from build123d import *

# Parameters (mm, degrees)
SKETCH1_W           = 304.8
SKETCH1_H           = 304.8
SKETCH1_R           = 6.3627
SKETCH1_R_2         = 1.778
SKETCH1_R_3         = 1.524
SKETCH1_R_4         = 1.190625
SKETCH1_W_2         = 10.0000054
SKETCH1_H_2         = 18.9999874
SKETCH1_W_3         = 71.12
SKETCH1_H_3         = 18.415
BOSS_EXTRUDE1_DEPTH = 2.54


with BuildPart() as part:
    # Sketch1 → Boss-Extrude1 (new body)
    with BuildSketch(Plane(origin=(0, 0, 0), x_dir=(1, 0, 0), z_dir=(0, 1, 0))):
        Rectangle(SKETCH1_W, SKETCH1_H)
        with Locations(Location((-133.35, 133.35, 0), (0, 0, 270))):
            Circle(SKETCH1_R, mode=Mode.SUBTRACT)
        with Locations(Location((-114.3, 133.35, 0), (0, 0, 270))):
            Circle(SKETCH1_R, mode=Mode.SUBTRACT)
        with Locations(Location((-95.25, 133.35, 0), (0, 0, 270))):
            Circle(SKETCH1_R, mode=Mode.SUBTRACT)
        with Locations(Location((-76.2, 133.35, 0), (0, 0, 270))):
            Circle(SKETCH1_R, mode=Mode.SUBTRACT)
        with Locations(Location((-57.15, 133.35, 0), (0, 0, 270))):
            Circle(SKETCH1_R, mode=Mode.SUBTRACT)
        with Locations(Location((-38.1, 133.35, 0), (0, 0, 270))):
            Circle(SKETCH1_R, mode=Mode.SUBTRACT)
        with Locations(Location((-19.05, 133.35, 0), (0, 0, 270))):
            Circle(SKETCH1_R, mode=Mode.SUBTRACT)
        with Locations(Location((0, 133.35, 0), (0, 0, 270))):
            Circle(SKETCH1_R, mode=Mode.SUBTRACT)
        with Locations(Location((19.05, 133.35, 0), (0, 0, 270))):
            Circle(SKETCH1_R, mode=Mode.SUBTRACT)
        with Locations(Location((38.1, 133.35, 0), (0, 0, 270))):
            Circle(SKETCH1_R, mode=Mode.SUBTRACT)
        with Locations(Location((57.15, 133.35, 0), (0, 0, 270))):
            Circle(SKETCH1_R, mode=Mode.SUBTRACT)
        with Locations(Location((76.2, 133.35, 0), (0, 0, 270))):
            Circle(SKETCH1_R, mode=Mode.SUBTRACT)
        with Locations(Location((95.25, 133.35, 0), (0, 0, 270))):
            Circle(SKETCH1_R, mode=Mode.SUBTRACT)
        with Locations(Location((114.3, 133.35, 0), (0, 0, 270))):
            Circle(SKETCH1_R, mode=Mode.SUBTRACT)
        with Locations(Location((133.35, 133.35, 0), (0, 0, 270))):
            Circle(SKETCH1_R, mode=Mode.SUBTRACT)
        with Locations(Location((-114.3, 0, 0), (0, 0, 270))):
            Circle(SKETCH1_R, mode=Mode.SUBTRACT)
        with Locations(Location((-95.25, 0, 0), (0, 0, 270))):
            Circle(SKETCH1_R, mode=Mode.SUBTRACT)
        with Locations(Location((-76.2, 0, 0), (0, 0, 270))):
            Circle(SKETCH1_R, mode=Mode.SUBTRACT)
        with Locations(Location((-57.15, 0, 0), (0, 0, 270))):
            Circle(SKETCH1_R, mode=Mode.SUBTRACT)
        with Locations(Location((-38.1, 0, 0), (0, 0, 270))):
            Circle(SKETCH1_R, mode=Mode.SUBTRACT)
        with Locations(Location((-19.05, 0, 0), (0, 0, 270))):
            Circle(SKETCH1_R, mode=Mode.SUBTRACT)
        with Locations(Location((0, 0, 0), (0, 0, 270))):
            Circle(SKETCH1_R, mode=Mode.SUBTRACT)
        with Locations(Location((-127.770384182, 146.820384182, 0), (0, 0, 270))):
            Circle(SKETCH1_R_2, mode=Mode.SUBTRACT)
        with Locations(Location((-100.829615818, 146.820384182, 0), (0, 0, 270))):
            Circle(SKETCH1_R_2, mode=Mode.SUBTRACT)
        with Locations(Location((-100.829615818, 119.879615818, 0), (0, 0, 270))):
            Circle(SKETCH1_R_2, mode=Mode.SUBTRACT)
        with Locations(Location((-127.770384182, 119.879615818, 0), (0, 0, 270))):
            Circle(SKETCH1_R_2, mode=Mode.SUBTRACT)
        with Locations(Location((-13.470384182, 146.820384182, 0), (0, 0, 270))):
            Circle(SKETCH1_R_2, mode=Mode.SUBTRACT)
        with Locations(Location((13.470384182, 146.820384182, 0), (0, 0, 270))):
            Circle(SKETCH1_R_2, mode=Mode.SUBTRACT)
        with Locations(Location((-114.3, -133.35, 0), (0, 0, 270))):
            Circle(SKETCH1_R, mode=Mode.SUBTRACT)
        with Locations(Location((-95.25, -133.35, 0), (0, 0, 270))):
            Circle(SKETCH1_R, mode=Mode.SUBTRACT)
        with Locations(Location((-76.2, -133.35, 0), (0, 0, 270))):
            Circle(SKETCH1_R, mode=Mode.SUBTRACT)
        with Locations(Location((-57.15, -133.35, 0), (0, 0, 270))):
            Circle(SKETCH1_R, mode=Mode.SUBTRACT)
        with Locations(Location((-38.1, -133.35, 0), (0, 0, 270))):
            Circle(SKETCH1_R, mode=Mode.SUBTRACT)
        with Locations(Location((-19.05, -133.35, 0), (0, 0, 270))):
            Circle(SKETCH1_R, mode=Mode.SUBTRACT)
        with Locations(Location((0, -133.35, 0), (0, 0, 270))):
            Circle(SKETCH1_R, mode=Mode.SUBTRACT)
        with Locations(Location((19.05, -133.35, 0), (0, 0, 270))):
            Circle(SKETCH1_R, mode=Mode.SUBTRACT)
        with Locations(Location((38.1, -133.35, 0), (0, 0, 270))):
            Circle(SKETCH1_R, mode=Mode.SUBTRACT)
        with Locations(Location((57.15, -133.35, 0), (0, 0, 270))):
            Circle(SKETCH1_R, mode=Mode.SUBTRACT)
        with Locations(Location((76.2, -133.35, 0), (0, 0, 270))):
            Circle(SKETCH1_R, mode=Mode.SUBTRACT)
        with Locations(Location((95.25, -133.35, 0), (0, 0, 270))):
            Circle(SKETCH1_R, mode=Mode.SUBTRACT)
        with Locations(Location((114.3, -133.35, 0), (0, 0, 270))):
            Circle(SKETCH1_R, mode=Mode.SUBTRACT)
        with Locations(Location((133.35, -133.35, 0), (0, 0, 270))):
            Circle(SKETCH1_R, mode=Mode.SUBTRACT)
        with Locations(Location((-133.35, 0, 0), (0, 0, 270))):
            Circle(SKETCH1_R, mode=Mode.SUBTRACT)
        with Locations(Location((-133.35, -133.35, 0), (0, 0, 270))):
            Circle(SKETCH1_R, mode=Mode.SUBTRACT)
        with Locations(Location((13.470384182, 119.879615818, 0), (0, 0, 270))):
            Circle(SKETCH1_R_2, mode=Mode.SUBTRACT)
        with Locations(Location((-13.470384182, 119.879615818, 0), (0, 0, 270))):
            Circle(SKETCH1_R_2, mode=Mode.SUBTRACT)
        with Locations(Location((127.770384182, 146.820384182, 0), (0, 0, 270))):
            Circle(SKETCH1_R_2, mode=Mode.SUBTRACT)
        with Locations(Location((127.770384182, 119.879615818, 0), (0, 0, 270))):
            Circle(SKETCH1_R_2, mode=Mode.SUBTRACT)
        with Locations(Location((100.829615818, 119.879615818, 0), (0, 0, 270))):
            Circle(SKETCH1_R_2, mode=Mode.SUBTRACT)
        with Locations(Location((100.829615818, 146.820384182, 0), (0, 0, 270))):
            Circle(SKETCH1_R_2, mode=Mode.SUBTRACT)
        with Locations(Location((127.770384182, -119.879615818, 0), (0, 0, 270))):
            Circle(SKETCH1_R_2, mode=Mode.SUBTRACT)
        with Locations(Location((127.770384182, -146.820384182, 0), (0, 0, 270))):
            Circle(SKETCH1_R_2, mode=Mode.SUBTRACT)
        with Locations(Location((100.829615818, -146.820384182, 0), (0, 0, 270))):
            Circle(SKETCH1_R_2, mode=Mode.SUBTRACT)
        with Locations(Location((100.829615818, -119.879615818, 0), (0, 0, 270))):
            Circle(SKETCH1_R_2, mode=Mode.SUBTRACT)
        with Locations(Location((13.470384182, -119.879615818, 0), (0, 0, 270))):
            Circle(SKETCH1_R_2, mode=Mode.SUBTRACT)
        with Locations(Location((13.470384182, -146.820384182, 0), (0, 0, 270))):
            Circle(SKETCH1_R_2, mode=Mode.SUBTRACT)
        with Locations(Location((-13.470384182, -146.820384182, 0), (0, 0, 270))):
            Circle(SKETCH1_R_2, mode=Mode.SUBTRACT)
        with Locations(Location((-13.470384182, -119.879615818, 0), (0, 0, 270))):
            Circle(SKETCH1_R_2, mode=Mode.SUBTRACT)
        with Locations(Location((-127.770384182, -119.879615818, 0), (0, 0, 270))):
            Circle(SKETCH1_R_2, mode=Mode.SUBTRACT)
        with Locations(Location((-127.770384182, -146.820384182, 0), (0, 0, 270))):
            Circle(SKETCH1_R_2, mode=Mode.SUBTRACT)
        with Locations(Location((-100.829615818, -146.820384182, 0), (0, 0, 270))):
            Circle(SKETCH1_R_2, mode=Mode.SUBTRACT)
        with Locations(Location((-100.829615818, -119.879615818, 0), (0, 0, 270))):
            Circle(SKETCH1_R_2, mode=Mode.SUBTRACT)
        with Locations(Location((-63.5, 97.4725, 0), (0, 0, 270))):
            Circle(SKETCH1_R_3, mode=Mode.SUBTRACT)
        with Locations(Location((-63.5, 70.8025, 0), (0, 0, 270))):
            Circle(SKETCH1_R_3, mode=Mode.SUBTRACT)
        with Locations(Location((-144.4625, 133.35, 0), (0, 0, 270))):
            Circle(SKETCH1_R_2, mode=Mode.SUBTRACT)
        with Locations(Location((-144.4625, 34.925, 0), (0, 0, 270))):
            Circle(SKETCH1_R_2, mode=Mode.SUBTRACT)
        with Locations(Location((-63.5, 13.335, 0), (0, 0, 270))):
            Circle(SKETCH1_R_3, mode=Mode.SUBTRACT)
        with Locations(Location((-63.5, -13.335, 0), (0, 0, 270))):
            Circle(SKETCH1_R_3, mode=Mode.SUBTRACT)
        with Locations(Location((-144.4625, 49.2125, 0), (0, 0, 270))):
            Circle(SKETCH1_R_2, mode=Mode.SUBTRACT)
        with Locations(Location((-144.4625, -49.2125, 0), (0, 0, 270))):
            Circle(SKETCH1_R_2, mode=Mode.SUBTRACT)
        with Locations(Location((-63.5, -70.8025, 0), (0, 0, 270))):
            Circle(SKETCH1_R_3, mode=Mode.SUBTRACT)
        with Locations(Location((-63.5, -97.4725, 0), (0, 0, 270))):
            Circle(SKETCH1_R_3, mode=Mode.SUBTRACT)
        with Locations(Location((-144.4625, -34.925, 0), (0, 0, 270))):
            Circle(SKETCH1_R_2, mode=Mode.SUBTRACT)
        with Locations(Location((-144.4625, -133.35, 0), (0, 0, 270))):
            Circle(SKETCH1_R_2, mode=Mode.SUBTRACT)
        with Locations(Location((114.3, 88.7000004, 0), (0, 0, 270))):
            Circle(SKETCH1_R_4, mode=Mode.SUBTRACT)
        with Locations(Location((114.3, 63.6999996, 0), (0, 0, 270))):
            Circle(SKETCH1_R_4, mode=Mode.SUBTRACT)
        with Locations(Location((31.73843479, 0, 0), (0, 0, 270))):
            Circle(SKETCH1_R_2, mode=Mode.SUBTRACT)
        with Locations(Location((120.66156521, 0, 0), (0, 0, 270))):
            Circle(SKETCH1_R_2, mode=Mode.SUBTRACT)
        with Locations((114.3, 76.2)):
            Rectangle(SKETCH1_W_2, SKETCH1_H_2, mode=Mode.SUBTRACT)
        with Locations((76.2, 0)):
            Rectangle(SKETCH1_W_3, SKETCH1_H_3, mode=Mode.SUBTRACT)
    extrude(amount=BOSS_EXTRUDE1_DEPTH)


solid = part.part
CAD build for the part. Positions are in the model's coordinates, mm. Round coordinates to 2 decimals unless told otherwise and drop trailing zeros. Order: outer loops, then holes, each group sorted by start corner. A loop starts at its lowest first (then second) coordinate and runs counter-clockwise, first axis right, second up. Notation, with made-up numbers: M 33,44.5 L 51,44.5 A22 cw 51,62.5 Z; hole C -20,60.5 d3. An arc over 180 degrees is marked long. Use one line per item in the form item = value.
Q1. Saw through at D-D on y = 1.1. State how many separate pieces and enclosed holes the cut face has, then the cut area to 3 significant figures.
Recorded:
separate_pieces = 1
enclosed_holes = 80
area = 86,200 mm^2
Q2. Flat gauge pin, fed straight in: P1, Ø11.5, axis at x = 114.3, z = -133.35, coming from the +Y side. Where does the tip first touch, or does it go through?
Recorded:
P1 = through
Q3. Probe L1, parallel to Z at x = -56.5, y = 0.4; L2, parallel to Z at x = -136, y = 1.15; L3, parallel to X at y = 2.25, z = 7. List the from-to ranges inside material, lowest first.
Recorded:
L1 = -152.4 to -139.68, -127.02 to -6.33, 6.33 to 127.02, 139.68 to 152.4
L2 = -152.4 to -139.13, -127.57 to -5.78, 5.78 to 127.57, 139.13 to 152.4
L3 = -152.4 to 40.64, 111.76 to 152.4
Q4. Two-plate mould, pull along Z, no slides. Class faces 1 (the flat face through (-2, 2.54, -36)), 2 (the cylindrical face through (80.5, 1.25, -138.04)): +Z half, -Z half, draft (parallel to the pull), parting line (faces both ways), or undercut.
Recorded:
face_1 = draft
face_2 = undercut
Q5. Saw through at A-A on x = 133.35. Give the cut face in (y, z), then the cut area to 3 significant figures.
Recorded:
outline = M 0,-152.4 L 2.54,-152.4 L 2.54,-139.71 L 0,-139.71 Z; M 0,-126.99 L 2.54,-126.99 L 2.54,126.99 L 0,126.99 Z; M 0,139.71 L 2.54,139.71 L 2.54,152.4 L 0,152.4 Z
area = 710 mm^2
Q6. Saw through at B-B on z = -78.5. Give the cut face in (x, y).
Recorded:
outline = M -152.4,0 L 109.3,0 L 109.3,2.54 L -152.4,2.54 Z; M 119.3,0 L 152.4,0 L 152.4,2.54 L 119.3,2.54 Z
Q7. Saw through at C-C on x = -57.15. Give the cut face in (y, z), then the cut area to 3 significant figures.
Recorded:
outline = M 0,-152.4 L 2.54,-152.4 L 2.54,-139.71 L 0,-139.71 Z; M 0,-126.99 L 2.54,-126.99 L 2.54,-6.36 L 0,-6.36 Z; M 0,6.36 L 2.54,6.36 L 2.54,126.99 L 0,126.99 Z; M 0,139.71 L 2.54,139.71 L 2.54,152.4 L 0,152.4 Z
area = 677 mm^2
